The figure shows three views and two pictorial views of one solid part (mm, origin at its lowest corner). Answer the questions. Give positions to 0.01 mm unless a question says otherwise; leave off trailing zeros. Loops run counter-clockwise (first coordinate to the right, second up) from the corner with the lowest first, then second, coordinate; pieces in that order, holes last. Notation, with made-up numbers: M 46,-37.5 L 60,-37.5 A12 cw 60,-28.5 Z; hole C 14,23 d7. An arc over 180 degrees is marked long. Write item = value, one per line. Start each with the question number.
1. Section B-B on z = 9 is taken. Determine the outline of the cut face in (x, y), plus the area to 3 significant figures.
2. Section A-A on y = 9 is taken. Determine the outline of the cut face in (x, z), plus the area to 3 significant figures.
3. Consider L1, parallel to Y at x = 39.5, z = 8.75; L2, parallel to Z at x = 18, y = 8.5; L3, parallel to Y at x = 29, z = 10.5. Determine where each line is inside the solid, lowest interval first. Write a range as [from, to].
4. Flat-ended cylindrical pins translate along their axes: pin 1 Ø3 at (x, y) = (26.5, 16) entering from +Z; pin 2 Ø6 at (x, z) = (25.5, 13) entering from +Y. Find the tip coordinate at first contact, or state that the pin passes through.
5. Section D-D on x = 37.5 is taken. Determine the outline of the cut face in (y, z), plus the area to 3 significant figures.
6. Section C-C on x = 70.5 is taken. Determine the outline of the cut face in (y, z), plus the area to 3 significant figures.
7. The mould has two halves that part along Y. Classify the marked faces 1 and 2: released by +Y, released by -Y, zero draft, split by the parting line, or undercut.
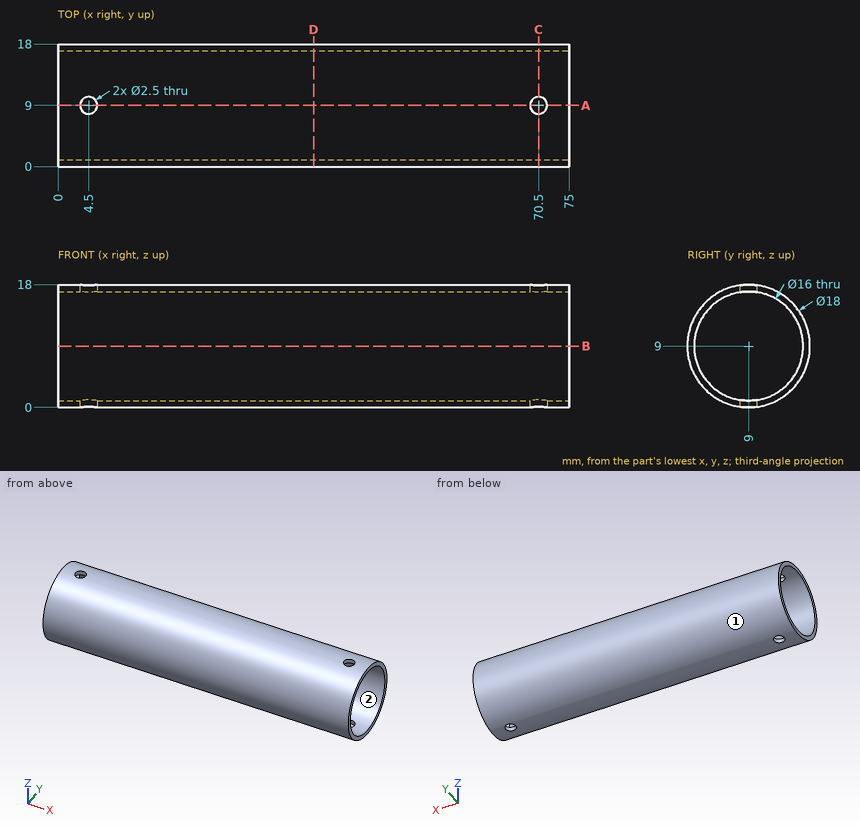
Verdict:
q1.outline = M 0,0 L 75,0 L 75,1 L 0,1 Z; M 0,17 L 75,17 L 75,18 L 0,18 Z
q1.area = 150 mm2
q2.outline = M 0,0 L 3.25,0 L 3.25,1 L 0,1 Z; M 0,17 L 3.25,17 L 3.25,18 L 0,18 Z; M 5.75,0 L 69.25,0 L 69.25,1 L 5.75,1 Z; M 5.75,17 L 69.25,17 L 69.25,18 L 5.75,18 Z; M 71.75,0 L 75,0 L 75,1 L 71.75,1 Z; M 71.75,17 L 75,17 L 75,18 L 71.75,18 Z
q2.area = 140 mm2
q3.L1 = [0, 1], [17, 18]
q3.L2 = [0.01, 1.02], [16.98, 17.99]
q3.L3 = [0.13, 1.14], [16.86, 17.87]
q4.pin_1 = 16.12
q4.pin_2 = 17.94
q5.outline = C 9,9 d18; hole C 9,9 d16
q5.area = 53.4 mm2
q6.outline = M 7.75,0.09 L 7.75,1.1 A8 cw 7.75,16.9 L 7.75,17.91 A9 ccw Z; M 10.25,0.09 A9 ccw 10.25,17.91 L 10.25,16.9 A8 cw 10.25,1.1 Z
q6.area = 48.4 mm2
q7.face_1 = split by the parting line
q7.face_2 = undercut
